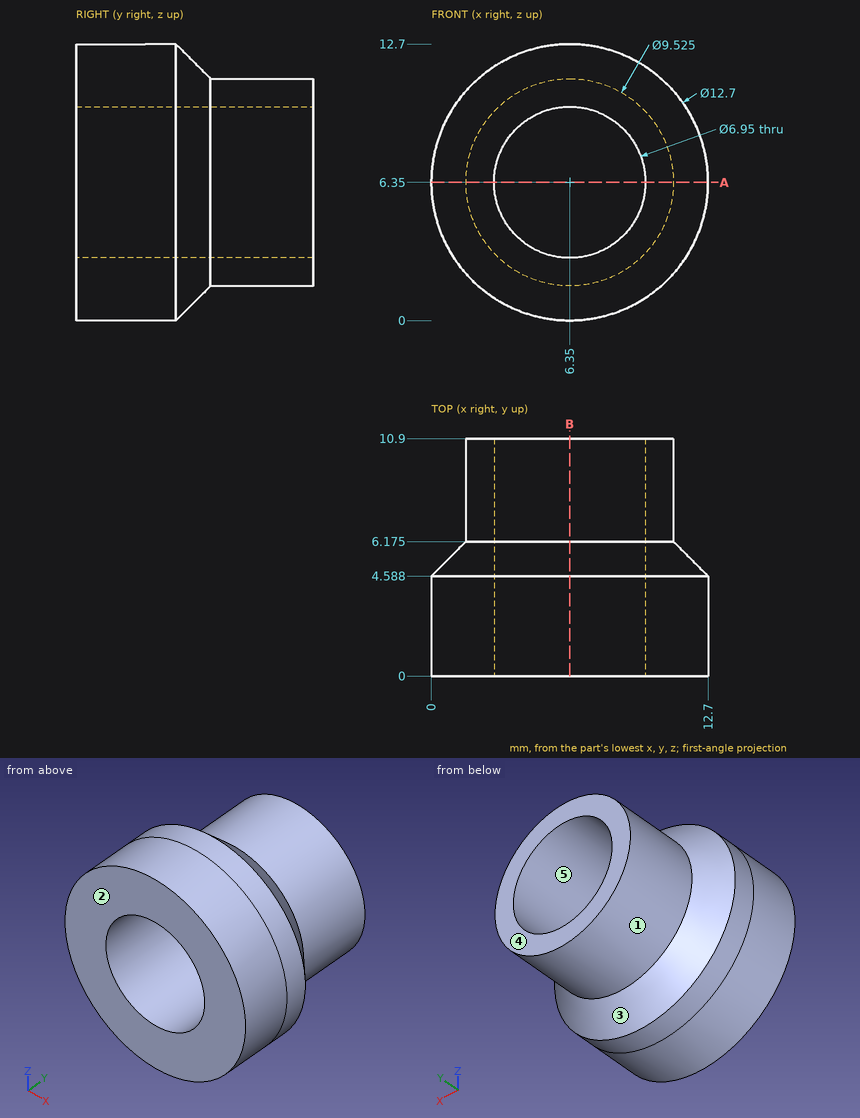
Geometry check sheet. Reference: drawing and pictorial views, mm from the part's lowest x, y, z. A direction names the side the tool comes from. Give positions to 0.01 mm unless a question says otherwise; leave off trailing zeros. Order: outer loops, then holes, each group sorted by start corner. A loop starts at its lowest first (then second) coordinate and runs counter-clockwise, first axis right, second up. Notation, with made-up numbers: (86.25, -33.5) - (143.25, -33.5) arc R25 ccw to (143.25, -5.5) - close; hole circle Ø8 at (8, 48.25). An arc over 180 degrees is marked (long way). Answer as CSV lines item,"result". Start each with the question number.
Item 1: Gauge pin test, flat ends, axial feed: pin 1 (5 mm diameter, centred on y = 8, z = 8, fed in from -X); pin 2 (6 mm diameter, centred on y = 10, z = 10.5, fed in from -X); pin 3 (1 mm diameter, centred on x = 11, y = 6, fed in from -Z) (1 decimal). Record the tip position at first contact, or that the pin passes through.
Item 2: Access from +Z, -Z, +X, -X, +Y, -Y to the whole of each face (thin tool, end or side, straight path). Record for the marked faces 1 and 2.
Item 3: Material ranges on L1, parallel to X at y = 8.75, z = 6.35 (1 decimal); L2, parallel to X at y = 2.5, z = 6.35 (1 decimal); L3, parallel to Z at x = 4.5, y = 10, recorded low to high.
Item 4: Section check B-B, the plane x = 6.35. Record the boundary of the cut face in (y, z) (1 decimal).
Item 5: Mould release check, pull along Z, two halves, no side actions. Record for the marked faces 3, 4 and 5: released by +Z, released by -Z, zero draft, split by the parting line, or undercut.
Item 6: Section check A-A, the plane z = 6.35. Record the boundary of the cut face in (x, y) (1 decimal).
Filled in:
1,pin 1,"x = 1.09"
1,pin 2,"x = 1.73"
1,pin 3,"z = 3.3"
2,face 1,"+Y"
2,face 2,"+Z, -Z, +X, -X, -Y"
3,L1,"1.6 to 2.9, 9.8 to 11.1"
3,L2,"0 to 2.9, 9.8 to 12.7"
3,L3,"1.96 to 3.41, 9.29 to 10.74"
4,outline,"(0, 0) - (4.6, 0) - (6.2, 1.6) - (10.9, 1.6) - (10.9, 2.9) - (0, 2.9) - close; (0, 9.8) - (10.9, 9.8) - (10.9, 11.1) - (6.2, 11.1) - (4.6, 12.7) - (0, 12.7) - close"
5,face 3,"split by the parting line"
5,face 4,"zero draft"
5,face 5,"undercut"
6,outline,"(0, 0) - (2.9, 0) - (2.9, 10.9) - (1.6, 10.9) - (1.6, 6.2) - (0, 4.6) - close; (9.8, 0) - (12.7, 0) - (12.7, 4.6) - (11.1, 6.2) - (11.1, 10.9) - (9.8, 10.9) - close"
